The listing builds one solid part. Answer for the finished solid, in the listing's coordinates (mm). A direction names the side the tool comes from. Coordinates: 2 decimals unless noted, no trailing zeros. Return JSON: item names as keys, results as strings. Group by question number.
1. Find the intervals of material crossed by line 1 along Y through (x, z) = (0, 18.5); line 2 along X through (y, z) = (0, 12.5); line 3 along Z through (x, y) = (1, -11), in increasing order.
2. The mould has two halves that part along X. Classify faces 3 (the face through (11, -7, 44.585)), 4 (the face through (0, 0, 1.309)): pulls with the +X half, pulls with the -X half, needs draft (parallel to the pull), parting line crosses it, or undercut.
3. Which of the six approach directions +Z, -Z, +X, -X, +Y, -Y give full straight-line access (tool end or side, diameter ignored) to faces 1 (the face through (0, 0, 0)), 2 (the face through (2.655, 11.955, 23.25))?
4. Each of these flat-tipped pins is pushed along its axis until it touches: P1, Ø6, axis at x = 6.5, z = 17.5, coming from the +Y side; P2, Ø1.5, axis at x = -9.5, z = 4.5, coming from the -Y side; P3, Ø6, axis at y = -6, z = 34.5, coming from the +X side. Where does it stop, or does it pass through?
Autodesk Fusion 360 part; units mm, degrees
sketch "Sketch1" plane through (0, 0, 0) normal (0, 0, 1) x (1, 0, 0)
  ellipse E0 centre (0, 0) end of major axis (0, 31.5965) minor radius 16.6986
  line L0 (0, -31.5965) -> (0, 31.5965)
  line L1 (16.6986, 0) -> (-16.6986, 0)
extrude "Extrude1" add sketch "Sketch1" along normal blind 44.585
ref_plane "WorkPlane1" through (0, 0, 13.758) normal (0, 0, 1) x (1, 0, 0)
sketch "Sketch9" plane through (0, 0, 44.585) normal (0, 0, 1) x (-1, 0, 0)
  circle A0 centre (0, 0) radius 12.2459
extrude "Extrude3" cut sketch "Sketch9" against normal blind 43.276
The answers:
{
 "1": {"line 1": "y = -31.6 to -12.25, 12.25 to 31.6", "line 2": "x = -16.7 to -12.25, 12.25 to 16.7", "line 3": "z = 0 to 1.31"},
 "2": {"face 3": "needs draft", "face 4": "undercut"},
 "3": {"face 1": "-Z, +X, -X, +Y, -Y", "face 2": "+Z"},
 "4": {"P1": "stops at y = 30.89", "P2": "stops at y = -26.91", "P3": "stops at x = 16.62"}
}
